Check sheet for the modelled part. Datum: model origin and axes. Units: mm. Give positions to 0.01 mm unless a question says otherwise; leave off trailing zeros. Write each loop counter-clockwise with the first axis right and the second up, starting at its lowest first coordinate (ties: lowest second). Pieces come first, ordered by that corner, then holes. Notation, with made-up numbers: M 5.5,43 L 45.5,43 A13 cw 45.5,55 Z; hole C 63,-29.5 d8. An arc over 180 degrees is marked long. One line per item, written item: value. Start each with the question number.
from build123d import *

# Parameters (mm, degrees)
SKETCH1_W           = 65
SKETCH1_H           = 58
SKETCH1_R           = 2.5
BOSS_EXTRUDE1_DEPTH = 36.33
SKETCH2_R           = 17.825
CUT_EXTRUDE1_DEPTH  = 80.911631819


with BuildPart() as part:
    # Sketch1 → Boss-Extrude1 (new body)
    with BuildSketch(Plane(origin=(0, 0, 0), x_dir=(1, 0, 0), z_dir=(0, 1, 0))):
        Rectangle(SKETCH1_W, SKETCH1_H)
        with Locations(Location((-16.25, 25, 0), (0, 0, 270))):
            Circle(SKETCH1_R, mode=Mode.SUBTRACT)
        with Locations(Location((16.25, 25, 0), (0, 0, 270))):
            Circle(SKETCH1_R, mode=Mode.SUBTRACT)
        with Locations(Location((16.25, -25, 0), (0, 0, 90))):
            Circle(SKETCH1_R, mode=Mode.SUBTRACT)
        with Locations(Location((-16.25, -25, 0), (0, 0, 90))):
            Circle(SKETCH1_R, mode=Mode.SUBTRACT)
        with Locations(Location((0, 25, 0), (0, 0, 270))):
            Circle(SKETCH1_R, mode=Mode.SUBTRACT)
        with Locations(Location((0, -25, 0), (0, 0, 270))):
            Circle(SKETCH1_R, mode=Mode.SUBTRACT)
    extrude(amount=BOSS_EXTRUDE1_DEPTH)

    # Sketch2 → Cut-Extrude1 (cut, through all)
    with BuildSketch(Plane(origin=(32.5, 0, 0), x_dir=(0, 0, -1), z_dir=(1, 0, 0))):
        with Locations((0, 36.33)):
            Circle(SKETCH2_R)
    extrude(amount=-CUT_EXTRUDE1_DEPTH, mode=Mode.SUBTRACT)


solid = part.part
1) Gauge pin test, flat ends, axial feed: pin 1 (6.5 mm diameter, centred on x = 0, z = 25, fed in from -Y); pin 2 (10 mm diameter, centred on x = -21.5, z = 6, fed in from +Y); pin 3 (12 mm diameter, centred on x = -5.5, z = 10, fed in from +Y). Record the tip position at first contact, or that the pin passes through.
2) Material ranges on L1, parallel to X at y = 20, z = 25; L2, parallel to Z at x = 16, y = 10; L3, parallel to Z at x = 1.5, y = 35.5, recorded low to high. Write a range as from..to.
3) Cross-section at C-C (z = -25). Record the boundary of the cut face in (x, y), plus the area to 3 significant figures.
4) Cross-section at D-D (y = 8.5). Record the boundary of the cut face in (x, z).
5) Draft check along Z on faces 1 (the flat face through (0, 36.33, 22)), 2 (the flat face through (0, 18, 29)), 3 (the flat face through (0, 18, -29)), 4 (the cylindrical face through (16.36, 17.911, -27.498)). Enter one of: released by +Z, released by -Z, zero draft, split by the parting line, or undercut.
6) Cross-section at B-B (y = 31). Record the boundary of the cut face in (x, z).
7) Cross-section at A-A (x = 1.5). Record the boundary of the cut face in (y, z) (3 decimals).
Data:
1. pin 1: stops at y = 0
1. pin 2: stops at y = 22.3
1. pin 3: stops at y = 28.47
2. L1: x = -32.5..-18.75, -13.75..-2.5, 2.5..13.75, 18.75..32.5
2. L2: z = -29..-27.49, -22.51..22.51, 27.49..29
2. L3: z = -29..-27, -23..-17.81, 17.81..23, 27..29
3. outline: M -32.5,0 L -18.75,0 L -18.75,36.33 L -32.5,36.33 Z; M -13.75,0 L -2.5,0 L -2.5,36.33 L -13.75,36.33 Z; M 2.5,0 L 13.75,0 L 13.75,36.33 L 2.5,36.33 Z; M 18.75,0 L 32.5,0 L 32.5,36.33 L 18.75,36.33 Z
3. area: 1,820 mm2
4. outline: M -32.5,-29 L 32.5,-29 L 32.5,29 L -32.5,29 Z; hole C -16.25,-25 d5; hole C -16.25,25 d5; hole C 0,-25 d5; hole C 0,25 d5; hole C 16.25,-25 d5; hole C 16.25,25 d5
5. face 1: zero draft
5. face 2: released by +Z
5. face 3: released by -Z
5. face 4: undercut
6. outline: M -32.5,-29 L 32.5,-29 L 32.5,-17.01 L -32.5,-17.01 Z; M -32.5,17.01 L 32.5,17.01 L 32.5,29 L -32.5,29 Z; hole C -16.25,-25 d5; hole C -16.25,25 d5; hole C 0,-25 d5; hole C 0,25 d5; hole C 16.25,-25 d5; hole C 16.25,25 d5
7. outline: M 0,-29 L 36.33,-29 L 36.33,-27 L 0,-27 Z; M 0,-23 L 36.33,-23 L 36.33,-17.825 A17.825 cw 36.33,17.825 L 36.33,23 L 0,23 Z; M 0,27 L 36.33,27 L 36.33,29 L 0,29 Z
